from build123d import *

# Parameters (mm, degrees)
SKETCH1_R           = 10.795
BOSS_EXTRUDE2_DEPTH = 3.175


with BuildPart() as part:
    # Sketch1 → Boss-Extrude2 (new body)
    with BuildSketch(Plane(origin=(0, 0, 0), x_dir=(1, 0, 0), z_dir=(0, 1, 0))):
        with BuildLine():
            Line((-58.904577704, 26.061934921), (-58.904577704, -26.061934921))
            ThreePointArc((-58.904577704, -26.061934921), (-69.399245848, -38.568993385), (-83.538673988, -30.405590742))
            ThreePointArc((-83.538673988, -30.405590742), (-88.9, 0), (-83.538673988, 30.405590742))
            ThreePointArc((-83.538673988, 30.405590742), (-69.399245848, 38.568993385), (-58.904577704, 26.061934921))
        make_face()
        with Locations((-76.2, 0)):
            Circle(SKETCH1_R, mode=Mode.SUBTRACT)
    extrude(amount=BOSS_EXTRUDE2_DEPTH)


solid = part.part
Part model, mm, in its own coordinate system. Coordinates: 2 decimals unless noted, no trailing zeros. Order: outer loops, then holes, each group sorted by start corner. A loop starts at its lowest first (then second) coordinate and runs counter-clockwise, first axis right, second up. Notation, with made-up numbers: M -31.5,-10.75 L -22.5,-10.75 A25 ccw -22.5,1.25 Z; hole C -1,87 d7. An arc over 180 degrees is marked long. One line per question, with ' | ' between items.
Q1. Drill centre lines: line 1 (Z direction, x = -76.2, y = 0.9) (3 decimals); line 2 (Z direction, x = -67, y = 1.15); line 3 (Z direction, x = -63.75, y = 0.5). Where is each one in solid material? Low to high.
A:
line 1: z = -37.901 to -10.795, 10.795 to 37.901 | line 2: z = -37.9 to -5.65, 5.65 to 37.9 | line 3: z = -36.04 to 36.04
Q2. Slice it at C-C (y = 2.3). Give the cut face in (x, z) (3 decimals), and give its area (3 significant figures).
A:
outline: M -83.539,-30.406 A12.7 ccw -58.905,-26.062 L -58.905,26.062 A12.7 ccw -83.539,30.406 A88.9 ccw Z; hole C -76.2,0 d21.59 | area: 1,640 mm^2
Q3. Slice it at A-A (z = 0). Give the cut face in (x, y) (3 decimals).
A:
outline: M -88.9,0 L -86.995,0 L -86.995,3.175 L -88.9,3.175 Z; M -65.405,0 L -58.905,0 L -58.905,3.175 L -65.405,3.175 Z
Q4. Slice it at D-D (z = -15). Give the cut face in (x, y) (3 decimals).
A:
outline: M -87.625,0 L -58.905,0 L -58.905,3.175 L -87.625,3.175 Z
Q5. Slice it at B-B (x = -76). Give the cut face in (y, z) (3 decimals), and give its area (3 significant figures).
A:
outline: M 0,-37.977 L 3.175,-37.977 L 3.175,-10.793 L 0,-10.793 Z; M 0,10.793 L 3.175,10.793 L 3.175,37.977 L 0,37.977 Z | area: 173 mm^2
Q6. Two-plate mould, pull along Z, no slides. Class faces 1 (the face through (-69.64, 1.57, -38.61)), 2 (the face through (-58.905, 2, 0)), 3 (the face through (-86.985, 1.565, -0.475)): +Z half, -Z half, draft (parallel to the pull), parting line (faces both ways), or undercut.
A:
face 1: -Z half | face 2: draft | face 3: undercut
Q7. Pin check, flat tip, straight feed: P1, Ø1, axis at x = -81.5, y = 0.5, coming from the -Z side. Stop position of the tip, or through.
A:
P1: stops at z = -34.61
